Autodesk Inventor part; units mm, degrees
ref_plane "YZ Plane" through (0, 0, 0) normal (1, 0, 0) x (0, 1, 0)
ref_plane "XZ Plane" through (0, 0, 0) normal (0, 1, 0) x (-1, 0, 0)
ref_plane "XY Plane" through (0, 0, 0) normal (0, 0, 1) x (1, 0, 0)
sketch "Skizze1" plane through (0, 0, 0) normal (1, 0, 0) x (0, 1, 0)
  line L0 (10, 45) -> (-10, 45)
  line L1 (-10, 45) -> (-10, -45)
  line L2 (-10, -45) -> (10, -45)
  line L3 (10, -45) -> (10, 45)
  line L4 (10, 45) -> (-10, -45) construction
  line L5 (-10, 45) -> (10, -45) construction
  point P0 (0, 0)
  dimension "d0" = 90
  dimension "d1" = 20
extrude "Extrusion1" add sketch "Skizze1" along normal blind 10
sketch "Skizze2" plane through (10, 0, 0) normal (1, 0, 0) x (0, 0, -1)
  line L0 (-45, 10) -> (-45, -10)
  point P0 (0, 0)
  point P1 (-35, 0)
  point P2 (35, 0)
  dimension "d4" = 10
  dimension "d5" = 70
hole "Bohrung1" at (10, 0, 35) at (10, 0, -35) direction (-1, 0, 0) diameter 4.5 end through all
fillet "Rundung1" radius 4 4 edges at (5, 10, 45) (5, -10, 45) (5, -10, -45) (5, 10, -45)
properties part number "103.019.01_Distanz_Wand"
CAD build for the part. Positions are in the model's coordinates, mm. Round coordinates to 2 decimals unless told otherwise and drop trailing zeros. Write each loop counter-clockwise with the first axis right and the second up, starting at its lowest first coordinate (ties: lowest second). Pieces come first, ordered by that corner, then holes. Notation, with made-up numbers: M -29.5,50.5 L 1.5,50.5 A13 cw 1.5,75.5 Z; hole C 18.25,-16 d3. An arc over 180 degrees is marked long. Put each result on its own line as item: value. Start each with the question number.
1) Pin check, flat tip, straight feed: pin 1 Ø1.5 at (y, z) = (-0.5, 34) entering from +X. Stop position of the tip, or through.
2) Drill centre lines: probe 1 along Z at (x, y) = (6.5, 0); probe 2 along Y at (x, z) = (6, -35); probe 3 along Z at (x, y) = (8.25, 1.75). Where is each one in solid material? Low to high. Write a range as [from, to].
3) Saw through at B-B, the plane z = -35. Write the cut outline in (x, y), and give its area (3 significant figures).
4) Saw through at C-C, the plane x = 8.5. Write the cut outline in (y, z), and give its area (3 significant figures).
5) Saw through at A-A, the plane y = 0. Write the cut outline in (x, z), and give its area (3 significant figures).
6) Pull direction Z, two halves, no side cores. Call faces 1 (the flat face through (5, 0, 45)), 2 (the cylindrical face through (5.07, 8.797, -43.859)), 3 (the cylindrical face through (4.93, 0.86, -37.08)), 4 (the cylindrical face through (4.93, 0.86, 32.92)): pulls with the +Z half, pulls with the -Z half, needs draft (parallel to the pull), parting line crosses it, or undercut.
Resolved:
1. pin 1: through
2. probe 1: [-45, -37.25], [-32.75, 32.75], [37.25, 45]
2. probe 2: [-10, -2.25], [2.25, 10]
2. probe 3: [-45, -36.41], [-33.59, 33.59], [36.41, 45]
3. outline: M 0,-10 L 10,-10 L 10,-2.25 L 0,-2.25 Z; M 0,2.25 L 10,2.25 L 10,10 L 0,10 Z
3. area: 155 mm²
4. outline: M -10,-41 A4 ccw -6,-45 L 6,-45 A4 ccw 10,-41 L 10,41 A4 ccw 6,45 L -6,45 A4 ccw -10,41 Z; hole C 0,-35 d4.5; hole C 0,35 d4.5
4. area: 1,750 mm²
5. outline: M 0,-45 L 10,-45 L 10,-37.25 L 0,-37.25 Z; M 0,-32.75 L 10,-32.75 L 10,32.75 L 0,32.75 Z; M 0,37.25 L 10,37.25 L 10,45 L 0,45 Z
5. area: 810 mm²
6. face 1: pulls with the +Z half
6. face 2: pulls with the -Z half
6. face 3: undercut
6. face 4: undercut
